```python
from build123d import *

# Parameters (mm, degrees)
SKETCH_1_W          = 100
SKETCH_1_H          = 100
EXTRUDE_1_DEPTH     = 10
CUT_EXTRUDE_1_DEPTH = 10
SKETCH_3_W          = 56.365102816
SKETCH_3_H          = 47.150770251
CUT_EXTRUDE_2_DEPTH = 9


with BuildPart() as part:
    # 草图1 → 凸台-拉伸1 (new body)
    with BuildSketch(Plane(origin=(0, 0, 0), x_dir=(1, 0, 0), z_dir=(0, 1, 0))):
        with Locations((-80.040161423, 118.55773228)):
            Rectangle(SKETCH_1_W, SKETCH_1_H)
        Polygon((-124.50987816, 163.027449017), (-124.50987816, 134.743177769), (-110.367742536, 148.885313393), align=None, mode=Mode.SUBTRACT)
        Polygon((-119.453493398, 164.389725441), (-104.604250993, 149.540483036), (-89.755008588, 164.389725441), align=None, mode=Mode.SUBTRACT)
        Polygon((-105.956547691, 144.474118548), (-121.512896877, 128.917769362), (-90.400198505, 128.917769362), align=None, mode=Mode.SUBTRACT)
        Polygon((-81.914917131, 162.05369475), (-98.178373098, 145.790238783), (-81.914917131, 129.526782816), align=None, mode=Mode.SUBTRACT)
    extrude(amount=EXTRUDE_1_DEPTH)

    # 草图2 → 切除-拉伸1 (cut)
    with BuildSketch(Plane(origin=(0, 10, 0), x_dir=(1, 0, 0), z_dir=(0, 1, 0))):
        Polygon((-130.040161423, 121.406962029), (-73.675058607, 121.406962029), (-73.675058607, 168.55773228), (-30.040161423, 168.55773228), (-30.040161423, 68.55773228), (-130.040161423, 68.55773228), align=None)
    extrude(amount=-CUT_EXTRUDE_1_DEPTH, mode=Mode.SUBTRACT)

    # 草图3 → 切除-拉伸2 (cut)
    with BuildSketch(Plane(origin=(0, 10, 0), x_dir=(1, 0, 0), z_dir=(0, 1, 0))):
        with Locations((-101.857610015, 144.982347155)):
            Rectangle(SKETCH_3_W, SKETCH_3_H)
    extrude(amount=-CUT_EXTRUDE_2_DEPTH, mode=Mode.SUBTRACT)


solid = part.part
```
The model under review builds one solid part; all positions refer to its coordinate system, in mm. A direction names the side the tool comes from. Give positions to 0.01 mm unless a question says otherwise; leave off trailing zeros. Write each loop counter-clockwise with the first axis right and the second up, starting at its lowest first coordinate (ties: lowest second). Pieces come first, ordered by that corner, then holes. Notation, with made-up numbers: M -18.5,15.25 L 18.5,15.25 A18 ccw 18.5,47.25 Z; hole C 42,13.25 d6. An arc over 180 degrees is marked long. Write each question's results on one line, items separated by ' | '. Start each with the question number.
1. We need section C-C (x = -93.5). Write out the cut boundary in (y, z), and give its area (3 significant figures).
2. We need section B-B (x = -86). Write out the cut boundary in (y, z).
3. We need section A-A (y = 0.3). Write out the cut boundary in (x, z) (1 decimal).
4. We need section D-D (z = -159.5). Write out the cut boundary in (x, y), and give its area (3 significant figures).
5. For faces 3 (the flat face through (-102, 1, -145)), 4 (the flat face through (-97.284, 0.493, -156.861)), list the 3-axis set-ups (+Z, -Z, +X, -X, +Y, -Y) from which the entire face can be reached by the end or side of a thin tool; tool diameter is ignored.
6. Mouldability with a two-part tool opening along Z and no side actions: class faces 1 (the flat face through (-102, 0, -145)), 2 (the flat face through (-98.07, 0.49, -136.59)) as released by +Z, released by -Z, zero draft, split by the parting line, or undercut.
7. For probe 1 along X at (y, z) = (0.95, -159.5); probe 2 along X at (y, z) = (0.2, -131.5); probe 3 along Z at (x, y) = (-114, 0.4), list the stretches that pass through material, from the lowest coordinate up. Write a range as [from, to].
Results found:
1) outline: M 0,-168.56 L 1,-168.56 L 1,-164.39 L 0,-164.39 Z; M 0,-160.64 L 1,-160.64 L 1,-150.47 L 0,-150.47 Z; M 0,-141.11 L 1,-141.11 L 1,-132.02 L 0,-132.02 Z; M 0,-128.92 L 1,-128.92 L 1,-121.41 L 0,-121.41 Z | area: 30.9 mm^2
2) outline: M 0,-168.56 L 1,-168.56 L 1,-157.97 L 0,-157.97 Z; M 0,-133.61 L 1,-133.61 L 1,-121.41 L 0,-121.41 Z
3) outline: M -130,-168.6 L -73.7,-168.6 L -73.7,-121.4 L -130,-121.4 Z; hole M -124.5,-163 L -110.4,-148.9 L -124.5,-134.7 Z; hole M -121.5,-128.9 L -106,-144.5 L -90.4,-128.9 Z; hole M -119.5,-164.4 L -89.8,-164.4 L -104.6,-149.5 Z; hole M -98.2,-145.8 L -81.9,-162.1 L -81.9,-129.5 Z
4) outline: M -130.04,0 L -124.51,0 L -124.51,1 L -130.04,1 Z; M -120.98,0 L -114.56,0 L -114.56,1 L -120.98,1 Z; M -94.64,0 L -84.47,0 L -84.47,1 L -94.64,1 Z; M -81.91,0 L -73.68,0 L -73.68,1 L -81.91,1 Z | area: 30.4 mm^2
5) face 3: +Z, -Z, +X, -X, +Y | face 4: +Y, -Y
6) face 1: zero draft | face 2: undercut
7) probe 1: x = [-130.04, -124.51], [-120.98, -114.56], [-94.64, -84.47], [-81.91, -73.68] | probe 2: x = [-130.04, -118.93], [-92.98, -83.89], [-81.91, -73.68] | probe 3: z = [-168.56, -164.39], [-158.94, -152.52], [-145.25, -136.43], [-128.92, -121.41]
